from build123d import *

# Parameters (mm, degrees)
CORTAR_EXTRUIR1_DEPTH = 2
CHAFL_N1_SIZE         = 0.5
REDONDEO1_R           = 0.5


with BuildPart() as part:
    # Croquis1 → Revolución1 (revolve)
    with BuildSketch(Plane.XY, mode=Mode.PRIVATE) as revoluci_n1_sk:
        Polygon((0, 0), (2.75, 0), (2.75, -3), (1.5, -3), (1.5, -43), (0, -43), align=None)
    revolve(revoluci_n1_sk.sketch.rotate(Axis((0, 0, 0), (0, -1, 0)), 90), axis=Axis((0, 0, 0), (0, -1, 0)))

    # Croquis2 → Cortar-Extruir1 (cut)
    with BuildSketch(Plane(origin=(0, 0, 0), x_dir=(1, 0, 0), z_dir=(0, 1, 0))):
        Polygon((1.25, 0.721687836), (0, 1.443375673), (-1.25, 0.721687836), (-1.25, -0.721687836), (0, -1.443375673), (1.25, -0.721687836), align=None)
    extrude(amount=-CORTAR_EXTRUIR1_DEPTH, mode=Mode.SUBTRACT)

    # Chaflán1
    chafl_n1_edges = [part.edges().sort_by_distance(p)[0] for p in [
        (0, -43, -1.5),
    ]]
    chamfer(chafl_n1_edges, length=CHAFL_N1_SIZE)

    # Redondeo1
    redondeo1_edges = [part.edges().sort_by_distance(p)[0] for p in [
        (0, 0, -2.75),
    ]]
    fillet(redondeo1_edges, radius=REDONDEO1_R)


solid = part.part
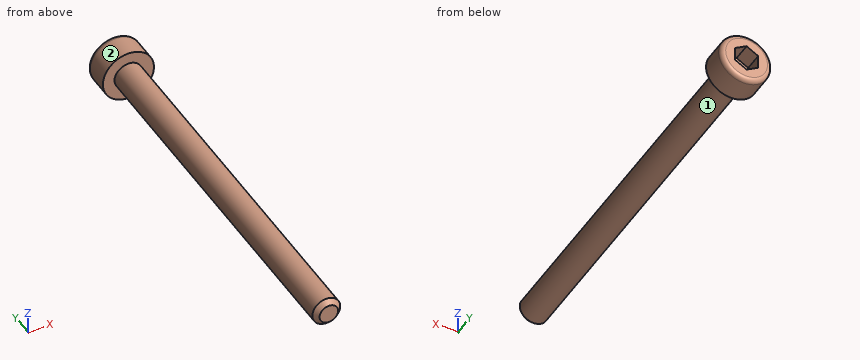
Model file for the job. Use its own axes, mm. Face numbers are marked on the shaded views. A direction names the side the tool comes from. Round coordinates to 2 decimals unless told otherwise and drop trailing zeros. Loops run counter-clockwise (first coordinate to the right, second up) from the corner with the lowest first, then second, coordinate; pieces in that order, holes last. Notation, with made-up numbers: (-0.5, 9.25) -> (44.5, 9.25) arc R16 ccw to (44.5, 22.25) -> close; hole circle Ø7 at (-16, 52). An arc over 180 degrees is marked (long way). Answer as CSV lines item,"result". Start each with the question number.
1) Probe line 1 along Z through (x, y) = (0.15, -32.5); line 2 along Y through (x, z) = (-0.6, 0.7); line 3 along Y through (x, z) = (1.85, -0.35). List the from-to ranges inside material, lowest first.
2) Pin check, flat tip, straight feed: P1, Ø1, axis at x = 1, y = -16, coming from the +Z side. Stop position of the tip, or through.
3) Tool access for the marked faces 1 and 2: list every direction of +Z, -Z, +X, -X, +Y, -Y with a clear straight run to the whole face (end or side of a thin tool).
4) Slice it at B-B (y = -6). List the corners of the cut face in (x, z).
5) Slice it at A-A (z = 0). List the corners of the cut face in (x, y), plus the area to 3 significant figures.
Filled in:
1,line 1,"z = -1.49 to 1.49"
1,line 2,"y = -43 to -2"
1,line 3,"y = -3 to 0"
2,P1,"stops at z = 1.41"
3,face 1,"-Y"
3,face 2,"+Y, -Y"
4,outline,"circle Ø3 at (0, 0)"
5,outline,"(-2.75, -3) -> (-1.5, -3) -> (-1.5, -42.5) -> (-1, -43) -> (1, -43) -> (1.5, -42.5) -> (1.5, -3) -> (2.75, -3) -> (2.75, -0.5) arc R0.5 ccw to (2.25, 0) -> (1.25, 0) -> (1.25, -2) -> (-1.25, -2) -> (-1.25, 0) -> (-2.25, 0) arc R0.5 ccw to (-2.75, -0.5) -> close"
5,area,"131 mm2"
